```python
from build123d import *

# Parameters (mm, degrees)
F0_W      = 700
F0_H      = 600
F0_R      = 25
F1_DEPTH  = 40
F2_R      = 30
F3_DEPTH  = 40
F5_DEPTH  = 20
F6_W      = 120
F6_H      = 60
F7_DEPTH  = 675
F8_W      = 440
F8_H      = 50
F9_DEPTH  = 60
F10_R     = 50
F10_R_2   = 25
F11_DEPTH = 5


with BuildPart() as f1:
    # F0 (on Front) → F1 (new body, symmetric)
    with BuildSketch(Plane.XZ):
        Rectangle(F0_W, F0_H)
        Circle(F0_R, mode=Mode.SUBTRACT)
    extrude(amount=F1_DEPTH, both=True)

    # F2 (on face) → F3 (cut)
    with BuildSketch(Plane(origin=(0, 40, 0), x_dir=(-1, 0, 0), z_dir=(0, 1, 0))):
        with Locations((-300, 0)):
            Circle(F2_R)
        with Locations((300, 0)):
            Circle(F2_R)
    extrude(amount=-F3_DEPTH, mode=Mode.SUBTRACT)

    # F4 (on face) → F5 (join)
    with BuildSketch(Plane.XZ.offset(40)):
        Polygon((-312.029017, -20.834869), (-287.970983, -20.834869), (-275.941965, 0), (-287.970983, 20.834869), (-312.029017, 20.834869), (-324.058035, 0), align=None)
        Polygon((287.970983, 20.834869), (275.941965, 0), (287.970983, -20.834869), (312.029017, -20.834869), (324.058035, 0), (312.029017, 20.834869), align=None)
    extrude(amount=F5_DEPTH)

    # F6 (on face) → F7 (join)
    with BuildSketch(Plane(origin=(0, 0, -300), x_dir=(1, 0, 0), z_dir=(0, 0, -1))):
        with Locations((-280, -0.602355)):
            Rectangle(F6_W, F6_H)
        with Locations((280, -0.602355)):
            Rectangle(F6_W, F6_H)
    extrude(amount=F7_DEPTH)

    # F8 (on face) → F9 (join)
    with BuildSketch(Plane.XZ.offset(29.397645)):
        with Locations((0, -755)):
            Rectangle(F8_W, F8_H)
    extrude(amount=-F9_DEPTH)

    # F10 (on face) → F11 (join)
    with BuildSketch(Plane.XZ.offset(40)):
        Circle(F10_R)
        Circle(F10_R_2, mode=Mode.SUBTRACT)
    extrude(amount=F11_DEPTH)


solid = f1.part
```
Part model, mm, in its own coordinate system. A direction names the side the tool comes from. Coordinates: 2 decimals unless noted, no trailing zeros. Write each loop counter-clockwise with the first axis right and the second up, starting at its lowest first coordinate (ties: lowest second). Pieces come first, ordered by that corner, then holes.
Item 1: Slice it at C-C (y = 13.5). Write the cut outline in (x, z).
Item 2: Slice it at A-A (x = -70). Write the cut outline in (y, z).
Item 3: Which spindle directions (+Z, -Z, +X, -X, +Y, -Y) get a long thin tool onto all of the face, cutting with end or side? Do faces 5 (the face through (222, -29.398, -633)), 6 (the face through (-22.9, -45, -10.4)), 7 (the face through (340, 1, -633)), 8 (the face through (-220, 1, -512)). Say none if no direction does.
Item 4: Pin check, flat tips, straight feed: pin 1 (6 mm diameter, centred on x = -296.5, y = -52, fed in from +Z); pin 2 (18 mm diameter, centred on y = -2.5, z = -695, fed in from +X); pin 3 (12 mm diameter, centred on y = 28, z = -367, fed in from -X). Stop position of each tip, or through.
Item 5: Slice it at B-B (z = -356). Write the cut outline in (x, y).
Item 6: Mould opens along X. For faces 1 (the face through (-220, 1, -876)), 2 (the face through (-340, 1, -633)), 3 (the face through (-3, 0, -780)), 4 (the face through (-5, -1, 300)) say: released by +X, released by -X, zero draft, split by the parting line, or undercut.
Item 7: Slice it at D-D (x = 0). Write the cut outline in (y, z).
Item 8: Probe line 1 (Z direction, x = 0, y = 6); line 2 (Z direction, x = 300, y = 16); line 3 (X direction, y = -27.5, z = 1.5). List the from-to ranges inside material, lowest first.
Results found:
1. outline: (-350, -300) - (-340, -300) - (-340, -975) - (-220, -975) - (-220, -780) - (220, -780) - (220, -975) - (340, -975) - (340, -300) - (350, -300) - (350, 300) - (-350, 300) - close; hole circle Ø60 at (-300, 0); hole (-220, -730) - (220, -730) - (220, -300) - (-220, -300) - close; hole circle Ø50 at (0, 0); hole circle Ø60 at (300, 0)
2. outline: (-40, -300) - (40, -300) - (40, 300) - (-40, 300) - close; (-29.4, -780) - (30.6, -780) - (30.6, -730) - (-29.4, -730) - close
3. face 5: -Z, +X, -X, -Y
3. face 6: +Z, -Z, -Y
3. face 7: -Z, +X, +Y, -Y
3. face 8: +Y, -Y
4. pin 1: stops at z = 20.83
4. pin 2: stops at x = 340
4. pin 3: stops at x = -340
5. outline: (-340, -29.4) - (-220, -29.4) - (-220, 30.6) - (-340, 30.6) - close; (220, -29.4) - (340, -29.4) - (340, 30.6) - (220, 30.6) - close
6. face 1: undercut
6. face 2: released by -X
6. face 3: undercut
6. face 4: zero draft
7. outline: (-45, -50) - (-40, -50) - (-40, -300) - (40, -300) - (40, -25) - (-45, -25) - close; (-45, 25) - (40, 25) - (40, 300) - (-40, 300) - (-40, 50) - (-45, 50) - close; (-29.4, -780) - (30.6, -780) - (30.6, -730) - (-29.4, -730) - close
8. line 1: z = -780 to -730, -300 to -25, 25 to 300
8. line 2: z = -975 to -30, 30 to 300
8. line 3: x = -350 to -24.95, 24.95 to 350
